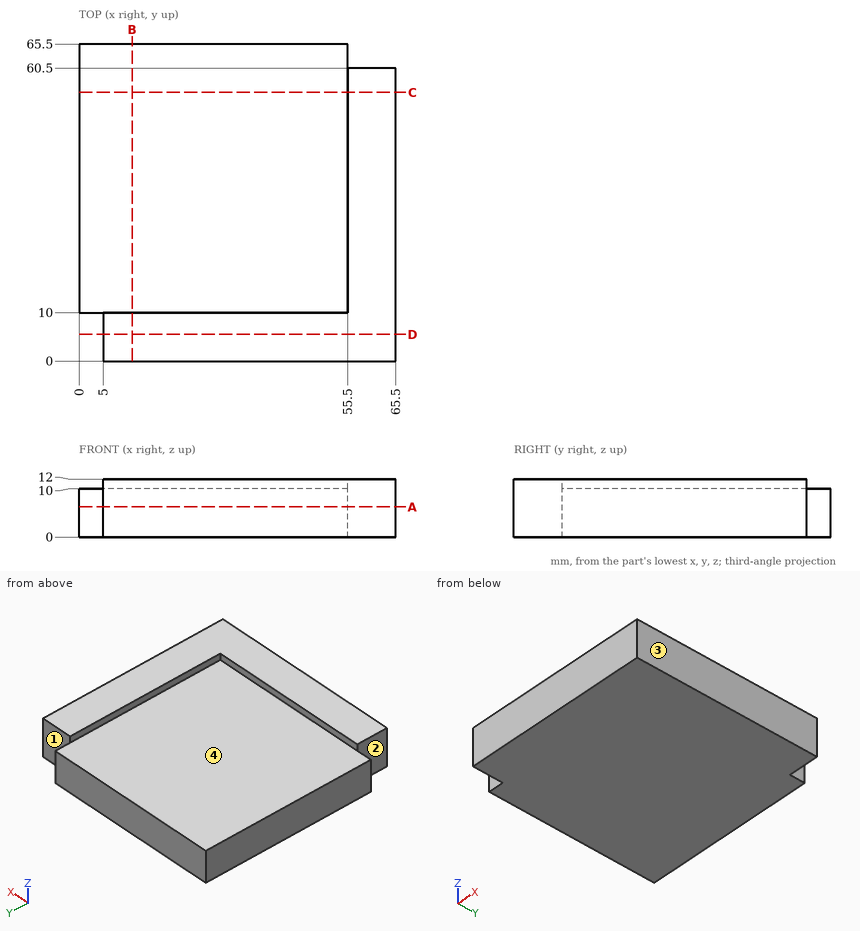
Part print with two shaded views. Sizes in mm from the minimum x, y, z corner. A direction names the side the tool comes from. Coordinates: 2 decimals unless noted, no trailing zeros. Write each loop counter-clockwise with the first axis right and the second up, starting at its lowest first coordinate (ties: lowest second). Pieces come first, ordered by that corner, then holes. Notation, with made-up numbers: M 10,39.5 L 30,39.5 A24 cw 30,66.5 Z; hole C 3.5,-24.5 d6. An arc over 180 degrees is marked long. Return JSON: item names as keys, results as strings.
Item 1: Slice it at D-D, the plane y = 5.5. Write the cut outline in (x, z).
Findings below:
{"outline": "M 5,0 L 65.5,0 L 65.5,12 L 5,12 Z"}
Item 2: Which spindle directions (+Z, -Z, +X, -X, +Y, -Y) get a long thin tool onto all of the face, cutting with end or side? Do the marked faces 1, 2, 3 and 4. Say none if no direction does.
Findings below:
{"face 1": "+Z, -Z, +X, +Y", "face 2": "+Z, -Z, -X, -Y", "face 3": "+Z, -Z, +X, +Y, -Y", "face 4": "+Z, -X, +Y"}
Item 3: Slice it at B-B, the plane x = 11. Write the cut outline in (y, z).
Findings below:
{"outline": "M 0,0 L 65.5,0 L 65.5,10 L 10,10 L 10,12 L 0,12 Z"}
Item 4: Slice it at C-C, the plane y = 55.5. Write the cut outline in (x, z).
Findings below:
{"outline": "M 0,0 L 65.5,0 L 65.5,12 L 55.5,12 L 55.5,10 L 0,10 Z"}
Item 5: Slice it at A-A, the plane z = 6.25. Write the cut outline in (x, y).
Findings below:
{"outline": "M 0,10 L 5,10 L 5,0 L 65.5,0 L 65.5,60.5 L 55.5,60.5 L 55.5,65.5 L 0,65.5 Z"}
Item 6: Drop flat-ended pins along their axis: pin 1 Ø1 at (x, z) = (28, 11) entering from +Y; pin 2 Ø4 at (x, y) = (45.5, 24) entering from +Z; pin 3 Ø5 at (x, z) = (58.5, 5.5) entering from +Y. Give the stop position or say it passes through.
Findings below:
{"pin 1": "stops at y = 10", "pin 2": "stops at z = 10", "pin 3": "stops at y = 60.5"}
Item 7: Probe line 1 (Z direction, x = 10.5, y = 61.5); line 2 (X direction, y = 44, z = 11); line 3 (Y direction, x = 61, z = 0.75). List the from-to ranges inside material, lowest first. Write a range as from..to.
Findings below:
{"line 1": "z = 0..10", "line 2": "x = 55.5..65.5", "line 3": "y = 0..60.5"}
